Study the drawing (mm; zero at the part's minimum x, y, z) and answer. A direction names the side the tool comes from. Coordinates: 2 decimals unless noted, no trailing zeros. Write each loop counter-clockwise with the first axis right and the second up, starting at its lowest first coordinate (ties: lowest second). Pieces come first, ordered by that corner, then holes. Notation, with made-up numbers: M 46.25,-35 L 90.25,-35 A26 ccw 90.25,-19 Z; hole C 51,50 d7. An arc over 180 degrees is marked long. Answer as CSV lines item,"result". Start each with the question number.
(1) The mould has two halves that part along Z. Classify the marked faces 4, 5 and 6: released by +Z, released by -Z, zero draft, split by the parting line, or undercut.
(2) A cutting plane is placed at D-D on z = 42. Give the vertices of the cut face in (x, y), then the cut area to 3 significant figures.
(3) A cutting plane is placed at B-B on x = 90.5. Give the vertices of the cut face in (y, z).
(4) Flat-ended cylindrical pins translate along their axes: P1, Ø20, axis at x = 88, y = 165.5, coming from the +Z side; P2, Ø25, axis at x = 30.5, z = 38, coming from the -Y side; P3, Ø16, axis at y = 294, z = 111.5, coming from the +X side. Find the tip coordinate at first contact, or state that the pin passes through.
(5) Find the intervals of material crossed by L1, parallel to Z at x = 86, y = 252; L2, parallel to Z at x = 41, y = 19.5; L3, parallel to Y at x = 92.5, z = 30.5, in increasing order. Write a range as [from, to].
(6) A cutting plane is placed at A-A on y = 25. Give the vertices of the cut face in (x, z), then the cut area to 3 significant figures.
(7) For the marked faces 1, 2 and 3, determine the directions among +Z, -Z, +X, -X, +Y, -Y from which every point of the face is accessible in a straight line to the end or side of a thin tool.
(8) A cutting plane is placed at C-C on y = 116. Give the vertices of the cut face in (x, z), then the cut area to 3 significant figures.
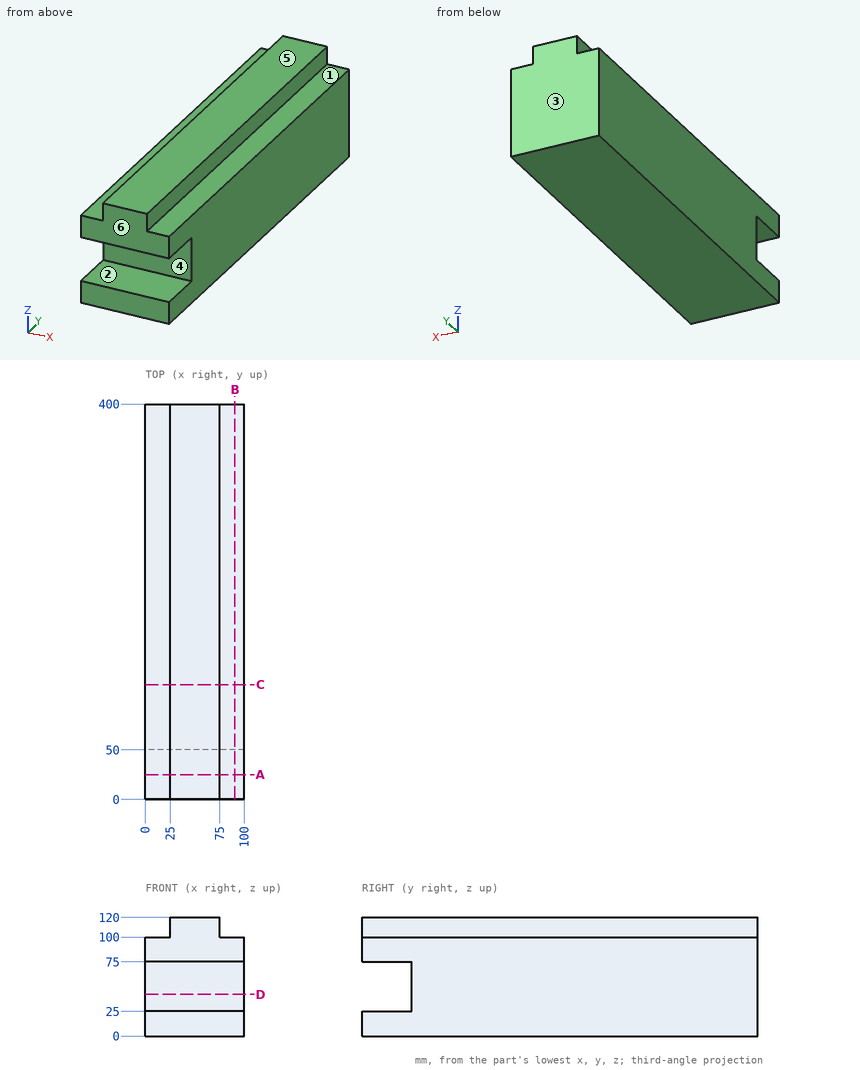
Here are the results:
1,face 4,"undercut"
1,face 5,"released by +Z"
1,face 6,"zero draft"
2,outline,"M 0,50 L 100,50 L 100,400 L 0,400 Z"
2,area,"35,000 mm^2"
3,outline,"M 0,0 L 400,0 L 400,100 L 0,100 L 0,75 L 50,75 L 50,25 L 0,25 Z"
4,P1,"stops at z = 100"
4,P2,"stops at y = 50"
4,P3,"stops at x = 75"
5,L1,"z = [0, 100]"
5,L2,"z = [0, 25], [75, 120]"
5,L3,"y = [50, 400]"
6,outline,"M 0,0 L 100,0 L 100,25 L 0,25 Z; M 0,75 L 100,75 L 100,100 L 75,100 L 75,120 L 25,120 L 25,100 L 0,100 Z"
6,area,"6,000 mm^2"
7,face 1,"+Z, +X, +Y, -Y"
7,face 2,"+X, -X, -Y"
7,face 3,"+Z, -Z, +X, -X, +Y"
8,outline,"M 0,0 L 100,0 L 100,100 L 75,100 L 75,120 L 25,120 L 25,100 L 0,100 Z"
8,area,"11,000 mm^2"
